```python
from build123d import *

# Parameters (mm, degrees)
F0_R          = 1.0795
F1_DEPTH      = 19.05
F3_DEPTH      = 50.8
F5_DEPTH      = 50.8
F7_DEPTH      = 50.8
F9_DEPTH      = 50.8
F11_DEPTH     = 50.8
F12_R         = 6.35
F13_T1_DEPTH  = 30.801632633
F13_T3_DEPTH  = 29.3245158286
F13_T5_DEPTH  = 29.3245158286
F13_T7_DEPTH  = 29.3245158286
F13_T9_DEPTH  = 29.3245158286
F13_T11_DEPTH = 29.3245158286


# Not quite as in the source:
# - a fillet or chamfer that OpenCascade refuses, or shapes differently, is made with other operations: its cross-section is extruded or revolved along the edge and cut away or added


with BuildPart() as f1:
    # F0 (on Top) → F1 (new body)
    with BuildSketch(Plane.XY):
        Polygon((-3.666268911, -11.1881585915), (9.5076317344, -6.9441600789), (9.5423084754, 6.8964316395), (-3.6101607654, 11.2063892332), (-11.7735105333, 0.0294977978), align=None)
        Circle(F0_R, mode=Mode.SUBTRACT)
    extrude(amount=F1_DEPTH)

    # F2 (on face) → F3 (join)
    with BuildSketch(Plane(origin=(-7.7198897222, -5.5793303969, 0), x_dir=(0.5857564721, -0.8104871099, 0), z_dir=(-0.8104871099, -0.5857564721, 0))):
        Polygon((6.9203175793, 19.05), (-6.9203175793, 0), (-2.9958017507, 0), (6.9203175793, 13.648367367), align=None)
    extrude(amount=F3_DEPTH)

    # F4 (on face) → F5 (join)
    with BuildSketch(Plane(origin=(2.9206814117, -9.0661593352, 0), x_dir=(0.9518277517, 0.3066332191, 0), z_dir=(0.3066332191, -0.9518277517, 0))):
        Polygon((6.9203175793, 19.05), (-6.9203175793, 0), (-2.9958017507, 0), (6.9203175793, 13.648367367), align=None)
    extrude(amount=F5_DEPTH)

    # F6 (on face) → F7 (join)
    with BuildSketch(Plane(origin=(9.5249701049, -0.0238642197, 0), x_dir=(0.0025054299, 0.9999968614, 0), z_dir=(0.9999968614, -0.0025054299, 0))):
        Polygon((6.9203175793, 19.05), (-6.9203175793, 0), (-2.9958017507, 0), (6.9203175793, 13.648367367), align=None)
    extrude(amount=F7_DEPTH)

    # F8 (on face) → F9 (join)
    with BuildSketch(Plane(origin=(2.966073855, 9.0514104363, 0), x_dir=(-0.9502793109, 0.3113988299, 0), z_dir=(0.3113988299, 0.9502793109, 0))):
        Polygon((6.9203175793, 19.05), (-6.9203175793, 0), (-2.9958017507, 0), (6.9203175793, 13.648367367), align=None)
    extrude(amount=F9_DEPTH)

    # F10 (on face) → F11 (join)
    with BuildSketch(Plane(origin=(-7.6918356494, 5.6179435155, 0), x_dir=(-0.5898103428, -0.8075418005, 0), z_dir=(-0.8075418005, 0.5898103428, 0))):
        Polygon((6.9203175793, 19.05), (-6.9203175793, 0), (-2.9958017507, 0), (6.9203175793, 13.648367367), align=None)
    extrude(amount=F11_DEPTH)

    # F12
    f12_edges = [f1.edges().sort_by_distance(p)[0] for p in [
        (-3.610161, 11.206389, 6.824184),
        (-11.773511, 0.029498, 6.824184),
        (-3.666269, -11.188159, 6.824184),
        (9.507632, -6.94416, 6.824184),
        (9.542308, 6.896432, 6.824184),
    ]]
    fillet(f12_edges, radius=F12_R)

    # F13: fillet of radius 5.08 on 10 edges, made by hand

    # F13_s2 → F13_t1 (cut)
    with BuildSketch(Plane.XY.offset(0.948367367)):
        with BuildLine():
            ThreePointArc((-49.800397455, 34.09417556), (-50.7175171639, 30.3158253164), (-48.6943216503, 26.9956266721))
            Line((-48.6943216503, 26.9956266721), (-52.7966339966, 29.9918632137))
            Line((-52.7966339966, 29.9918632137), (-49.800397455, 34.09417556))
        make_face()
        with BuildLine():
            ThreePointArc((-47.8146569743, -36.8273128564), (-44.5046379302, -38.8671199678), (-40.7217395774, -37.9689444966))
            Line((-40.7217395774, -37.9689444966), (-44.8390140959, -40.9445873749))
            Line((-44.8390140959, -40.9445873749), (-47.8146569743, -36.8273128564))
        make_face()
        with BuildLine():
            ThreePointArc((20.2493142845, -56.8547066196), (23.2121382661, -54.3370265013), (23.5269025104, -50.4617248879))
            Line((23.5269025104, -50.4617248879), (25.0845992633, -55.2970098667))
            Line((25.0845992633, -55.2970098667), (20.2493142845, -56.8547066196))
        make_face()
        with BuildLine():
            ThreePointArc((60.329421451, 1.6891717451), (58.8505283301, 5.2849907424), (55.2621649789, 6.7818833849))
            Line((55.2621649789, 6.7818833849), (60.3421490348, 6.769155801))
            Line((60.3421490348, 6.769155801), (60.329421451, 1.6891717451))
        make_face()
        with BuildLine():
            ThreePointArc((10.6269937385, 54.6531593275), (13.1594884979, 57.6033304103), (17.0363186938, 57.8986721709))
            Line((17.0363186938, 57.8986721709), (12.2088997945, 59.4805782269))
            Line((12.2088997945, 59.4805782269), (10.6269937385, 54.6531593275))
        make_face()
    extrude(amount=F13_T1_DEPTH, mode=Mode.SUBTRACT)

    # F13_s4 → F13_t3 (cut)
    with BuildSketch(Plane(origin=(11.5722662379, 15.8442265835, 0), x_dir=(0, 0, 1), z_dir=(-0.5898103428, -0.8075418005, 0))):
        with BuildLine():
            ThreePointArc((0, 55.245), (1.4878975516, 58.8371024484), (5.08, 60.325))
            Line((5.08, 60.325), (0, 60.325))
            Line((0, 60.325), (0, 55.245))
        make_face()
    extrude(amount=F13_T3_DEPTH, mode=Mode.SUBTRACT)

    # F13_s6 → F13_t5 (cut)
    with BuildSketch(Plane(origin=(-11.492728007, 15.9020144909, 0), x_dir=(0, 0, 1), z_dir=(0.5857564721, -0.8104871099, 0))):
        with BuildLine():
            ThreePointArc((0, 55.245), (1.4878975516, 58.8371024484), (5.08, 60.325))
            Line((5.08, 60.325), (0, 60.325))
            Line((0, 60.325), (0, 55.245))
        make_face()
    extrude(amount=F13_T5_DEPTH, mode=Mode.SUBTRACT)

    # F13_s8 → F13_t7 (cut)
    with BuildSketch(Plane(origin=(-18.6751627697, -6.0162411386, 0), x_dir=(0, 0, 1), z_dir=(0.9518277517, 0.3066332191, 0))):
        with BuildLine():
            ThreePointArc((0, 55.245), (1.4878975516, 58.8371024484), (5.08, 60.325))
            Line((5.08, 60.325), (0, 60.325))
            Line((0, 60.325), (0, 55.245))
        make_face()
    extrude(amount=F13_T7_DEPTH, mode=Mode.SUBTRACT)

    # F13_s10 → F13_t9 (cut)
    with BuildSketch(Plane(origin=(-0.0491573301, -19.620255999, 0), x_dir=(0, 0, 1), z_dir=(0.0025054299, 0.9999968614, 0))):
        with BuildLine():
            ThreePointArc((0, 55.245), (1.4878975516, 58.8371024484), (5.08, 60.325))
            Line((5.08, 60.325), (0, 60.325))
            Line((0, 60.325), (0, 55.245))
        make_face()
    extrude(amount=F13_T9_DEPTH, mode=Mode.SUBTRACT)

    # F13_s12 → F13_t11 (cut)
    with BuildSketch(Plane(origin=(18.6447818689, -6.1097439368, 0), x_dir=(0, 0, 1), z_dir=(-0.9502793109, 0.3113988299, 0))):
        with BuildLine():
            ThreePointArc((0, 55.245), (1.4878975516, 58.8371024484), (5.08, 60.325))
            Line((5.08, 60.325), (0, 60.325))
            Line((0, 60.325), (0, 55.245))
        make_face()
    extrude(amount=F13_T11_DEPTH, mode=Mode.SUBTRACT)


solid = f1.part
```
Could you check a few things on this model? Use its own coordinates, in mm. A direction names the side the tool comes from. Round coordinates to 2 decimals unless told otherwise and drop trailing zeros. Loops run counter-clockwise (first coordinate to the right, second up) from the corner with the lowest first, then second, coordinate; pieces in that order, holes last. Notation, with made-up numbers: M 53.5,7 L 63.5,7 A33 ccw 63.5,42 Z; hole C -11,79.5 d5. An arc over 180 degrees is marked long. Write item = value, one per line.
1. I want a section at A-A, the plane x = -37. Write out the boundary of the cut face in (y, z), and give its area (3 significant figures).
Results below:
outline = M -35.28,13.65 L -23.04,0 L -18.2,0 L -35.28,19.05 Z; M 18.45,13.65 L 30.73,0 L 35.59,0 L 18.45,19.05 Z
area = 159 mm²
2. I want a section at B-B, the plane y = -17.5. Write out the boundary of the cut face in (x, z), and give its area (3 significant figures).
Results below:
outline = M -36.03,0 L -29.33,0 L -12.4,13.65 L -12.4,19.05 Z; M -1.63,0 L 2.49,0 L 12.91,13.65 L 12.91,19.05 Z
area = 177 mm²
3. Which directions (+Z, -Z, +X, -X, +Y, -Y) give clear straight access to the entire face, cutting with the end or side of a thin tool? Please do faces 4 (the face through (-8.162, 4.975, 1.976)), 5 (the face through (-21.93, -24.39, 16.31)), 6 (the face through (3.68, -8.82, 1.98)).
Results below:
face_4 = -Z, -X
face_5 = +Z, -Z, -Y
face_6 = -Z, +X
4. I want a section at C-C, the plane y = 49. Write out the boundary of the cut face in (x, z), and give its area (3 significant figures).
Results below:
outline = M 8.77,13.65 L 19.21,0 L 23.34,0 L 8.77,19.05 Z
area = 67.5 mm²
5. I need wall thicknesses on probe 1 along X at (y, z) = (-19.5, 16.75); probe 2 along X at (y, z) = (-18, 13); probe 3 along Y at (x, z) = (-19.5, 18.25). Which ranges of each line are inside material? Lowest first, please.
Results below:
probe_1 = -18.02 to -15.17, 11.8 to 13.55
probe_2 = -20.6 to -13.9, 8.45 to 12.57
probe_3 = -22.63 to -21.91, 5.67 to 6.39
6. Will these pins go through, and if not, where does the flat tip stop? P1, Ø1, axis at x = 35, z = 4.5, coming from the +Y side; P2, Ø8, axis at x = -2, z = 3, coming from the +Y side; P3, Ø1, axis at x = 34, z = 15.5, coming from the +Y side; P4, Ø6, axis at x = 32.5, y = -8, coming from the -Z side.
Results below:
P1 = 0.55
P2 = 11.96
P3 = 6.84
P4 = 0
7. Thinking about a two-plate mould opening in X: for faces 1 (the face through (-45.115, 37.919, 1.449)), 2 (the face through (10.359, 31.924, 9.658)), 3 (the face through (-7.25, -6.23, 1.98)), which applies, +X half, -X half, draft (parallel to the pull), parting line (faces both ways), or undercut?
Results below:
face_1 = -X half
face_2 = +X half
face_3 = undercut
